The listing builds one solid part. Answer for the finished solid, in the listing's coordinates (mm). A direction names the side the tool comes from. Round coordinates to 2 decimals unless told otherwise and drop trailing zeros. Loops run counter-clockwise (first coordinate to the right, second up) from the corner with the lowest first, then second, coordinate; pieces in that order, holes last. Notation, with made-up numbers: (-17, 29.25) -> (1, 29.25) arc R10 cw to (1, 41.25) -> close; hole circle Ø4 at (46.25, 19). An arc over 180 degrees is marked (long way). Use a Markdown table: item, result. Add a question column.
Q1. Which of the six approach directions +Z, -Z, +X, -X, +Y, -Y give full straight-line access (tool end or side, diameter ignored) to faces 1 (the flat face through (7.85, 0, 1)), 2 (the cylindrical face through (5.03, -6.45, 1.08)), 3 (the flat face through (10, -7.5, 1))?
Q2. Section D-D on y = -8.25 is taken. Give the vertices of the cut face in (x, z).
Q3. Consider line 1 (Y direction, x = -1, z = 0.5); line 2 (X direction, y = -2.75, z = 1.4); line 3 (X direction, y = 3, z = 0.45). Determine where each line is inside the solid, lowest interval first.
Q4. Section A-A on x = 2.5 is taken. Give the vertices of the cut face in (y, z).
Q5. Section B-B on x = -5.05 is taken. Give the vertices of the cut face in (y, z).
Q6. Given pin 1 Ø1 at (x, y) = (1.5, 2.5) entering from -Z; pin 2 Ø0.7 at (y, z) = (-0.5, 0.5) entering from +X; pin 3 Ø5 at (x, y) = (-10.5, 4) entering from -Z; pin 4 Ø1.1 at (x, z) = (12.5, 0.5) entering from -Y, each flat-ended and moving along its own axis, determine where each tip first touches the part or whether it passes through.
Q7. For a pull along Y with two mould halves and no side action, classify faces 4 (the flat face through (0, -10.5, 1)), 5 (the flat face through (0, 4, 1)), 6 (the cylindrical face through (16.05, 7.07, 1.12)) as released by +Y, released by -Y, zero draft, split by the parting line, or undercut.
Q8. Section C-C on z = 1.6 is taken. Give the number of separate pieces and of enclosed holes in the cut face, then the cut area to 3 significant figures.
from build123d import *

# Parameters (mm, degrees)
SKETCH_1_R      = 1.55
SKETCH_1_W      = 15.7
SKETCH_1_H      = 7.5
EXTRUDE_1_DEPTH = 2.2
FILLET_1_R      = 2
FILLET_2_R      = 1.5
FILLET_3_R      = 2


with BuildPart() as part:
    # 草图1 → 凸台-拉伸1 (new body)
    with BuildSketch(Plane.XY):
        with BuildLine():
            ThreePointArc((-16.5, 3.968626967), (-21, 0), (-16.5, -3.968626967))
            Line((-16.5, -3.968626967), (-16.5, -7.5))
            Line((-16.5, -7.5), (-6.1, -7.5))
            ThreePointArc((-6.1, -7.5), (-5.05, -6.45), (-4, -7.5))
            Line((-4, -7.5), (-4, -10.5))
            Line((-4, -10.5), (4, -10.5))
            Line((4, -10.5), (4, -7.5))
            ThreePointArc((4, -7.5), (5.05, -6.45), (6.1, -7.5))
            Line((6.1, -7.5), (16.5, -7.5))
            Line((16.5, -7.5), (16.5, -3.968626967))
            ThreePointArc((16.5, -3.968626967), (21, 0), (16.5, 3.968626967))
            Line((16.5, 3.968626967), (16.5, 7.5))
            Line((16.5, 7.5), (-16.5, 7.5))
            Line((-16.5, 7.5), (-16.5, 3.968626967))
        make_face()
        with Locations((-17, 0)):
            Circle(SKETCH_1_R, mode=Mode.SUBTRACT)
        with BuildLine():
            Line((-14.15, 4.1), (-11.85, 4.1))
            ThreePointArc((-11.85, 4.1), (-11.10753788, 3.79246212), (-10.8, 3.05))
            ThreePointArc((-10.8, 3.05), (-11.10753788, 2.30753788), (-11.85, 2))
            Line((-11.85, 2), (-11.85, -2))
            ThreePointArc((-11.85, -2), (-11.10753788, -2.30753788), (-10.8, -3.05))
            ThreePointArc((-10.8, -3.05), (-11.10753788, -3.79246212), (-11.85, -4.1))
            Line((-11.85, -4.1), (-14.15, -4.1))
            ThreePointArc((-14.15, -4.1), (-15.2, -3.05), (-14.15, -2))
            Line((-14.15, -2), (-14.15, 2))
            ThreePointArc((-14.15, 2), (-15.2, 3.05), (-14.15, 4.1))
        make_face(mode=Mode.SUBTRACT)
        with Locations((0, 0.25)):
            Rectangle(SKETCH_1_W, SKETCH_1_H, mode=Mode.SUBTRACT)
        with BuildLine():
            Line((11.85, 4.1), (14.15, 4.1))
            ThreePointArc((14.15, 4.1), (14.89246212, 3.79246212), (15.2, 3.05))
            ThreePointArc((15.2, 3.05), (14.89246212, 2.30753788), (14.15, 2))
            Line((14.15, 2), (14.15, -2))
            ThreePointArc((14.15, -2), (14.89246212, -2.30753788), (15.2, -3.05))
            ThreePointArc((15.2, -3.05), (14.89246212, -3.79246212), (14.15, -4.1))
            Line((14.15, -4.1), (11.85, -4.1))
            ThreePointArc((11.85, -4.1), (10.8, -3.05), (11.85, -2))
            Line((11.85, -2), (11.85, 2))
            ThreePointArc((11.85, 2), (10.8, 3.05), (11.85, 4.1))
        make_face(mode=Mode.SUBTRACT)
        with Locations((17, 0)):
            Circle(SKETCH_1_R, mode=Mode.SUBTRACT)
    extrude(amount=EXTRUDE_1_DEPTH)

    # 圆角1
    fillet_1_edges = [part.edges().sort_by_distance(p)[0] for p in [
        (-16.5, -3.968626967, 1.1),
        (-16.5, 3.968626967, 1.1),
        (16.5, 3.968626967, 1.1),
        (16.5, -3.968626967, 1.1),
    ]]
    fillet(fillet_1_edges, radius=FILLET_1_R)

    # 圆角2
    fillet_2_edges = [part.edges().sort_by_distance(p)[0] for p in [
        (-16.5, -7.5, 1.1),
        (-16.5, 7.5, 1.1),
        (16.5, 7.5, 1.1),
        (16.5, -7.5, 1.1),
    ]]
    fillet(fillet_2_edges, radius=FILLET_2_R)

    # 圆角3
    fillet_3_edges = [part.edges().sort_by_distance(p)[0] for p in [
        (-7.85, -3.5, 1.1),
        (7.85, -3.5, 1.1),
        (7.85, 4, 1.1),
        (-7.85, 4, 1.1),
    ]]
    fillet(fillet_3_edges, radius=FILLET_3_R)


solid = part.part
Checked values:
| question | item | result |
|---|---|---|
| 1 | face 1 | +Z, -Z |
| 1 | face 2 | +Z, -Z, -Y |
| 1 | face 3 | +Z, -Z, +X, -Y |
| 2 | outline | (-4, 0) -> (4, 0) -> (4, 2.2) -> (-4, 2.2) -> close |
| 3 | line 1 | y = -10.5 to -3.5, 4 to 7.5 |
| 3 | line 2 | x = -19.9 to -15.16, -10.84 to -7.41, 7.41 to 10.84, 15.16 to 19.9 |
| 3 | line 3 | x = -19.65 to -15.2, -10.8 to -7.58, 7.58 to 10.8, 15.2 to 19.65 |
| 4 | outline | (-10.5, 0) -> (-3.5, 0) -> (-3.5, 2.2) -> (-10.5, 2.2) -> close; (4, 0) -> (7.5, 0) -> (7.5, 2.2) -> (4, 2.2) -> close |
| 5 | outline | (-6.45, 0) -> (-3.5, 0) -> (-3.5, 2.2) -> (-6.45, 2.2) -> close; (4, 0) -> (7.5, 0) -> (7.5, 2.2) -> (4, 2.2) -> close |
| 6 | pin 1 | passes through |
| 6 | pin 2 | stops at x = 21 |
| 6 | pin 3 | stops at z = 0 |
| 6 | pin 4 | stops at y = -7.5 |
| 7 | face 4 | released by -Y |
| 7 | face 5 | undercut |
| 7 | face 6 | released by +Y |
| 8 | separate pieces | 1 |
| 8 | enclosed holes | 5 |
| 8 | area | 393 mm2 |
